from build123d import *

# Parameters (mm, degrees)
SKETCH2_W           = 25
SKETCH2_H           = 25
SKETCH2_R           = 9.247
BOSS_EXTRUDE1_DEPTH = 100
BOSS_EXTRUDE1_DRAFT = -0.05
FILLET4_R           = 2


with BuildPart() as part:
    # Sketch2 → Boss-Extrude1 (with draft: the straight prism first)
    with BuildSketch(Plane(origin=(0, 0, 0), x_dir=(1, 0, 0), z_dir=(0, 1, 0))):
        Rectangle(SKETCH2_W, SKETCH2_H)
        Circle(SKETCH2_R, mode=Mode.SUBTRACT)
    extrude(amount=BOSS_EXTRUDE1_DEPTH)
    # Boss-Extrude1: the draft: its side faces are tilted about the plane it starts from
    boss_extrude1_sides = [part.faces().sort_by_distance(p)[0] for p in [
        (-12.5, 50, 0),
        (0, 50, 12.5),
        (12.5, 50, 0),
        (0, 50, -12.5),
        (-9.247, 50, 0),
    ]]
    draft(boss_extrude1_sides, Plane(origin=(0, 0, 0), x_dir=(1, 0, 0), z_dir=(0, 1, 0)), BOSS_EXTRUDE1_DRAFT)

    # Fillet4
    fillet4_edges = [part.edges().sort_by_distance(p)[0] for p in [
        (0, 0, 12.5),
        (-12.5, 0, 0),
        (0, 0, -12.5),
        (12.5, 0, 0),
        (-12.543633242, 50, -12.543633242),
        (12.543633242, 50, -12.543633242),
    ]]
    fillet(fillet4_edges, radius=FILLET4_R)


solid = part.part
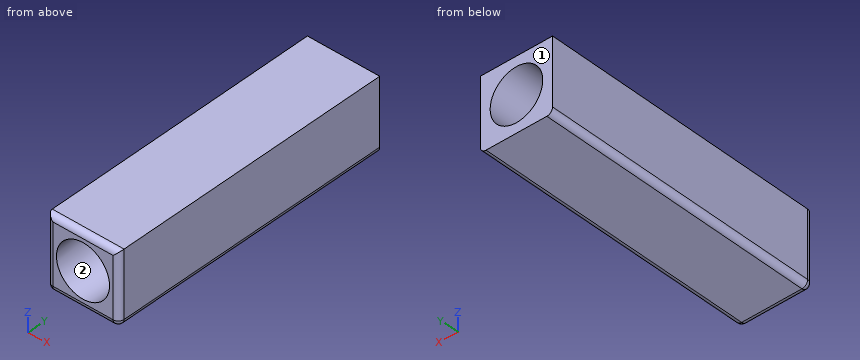
CAD build for the part. Positions are in the model's coordinates, mm. Face numbers are marked on the shaded views. Round coordinates to 2 decimals unless told otherwise and drop trailing zeros.
(1) Drop flat-ended pins along their axis: P1, Ø12, axis at x = -0.5, z = -2, coming from the +Y side; P2, Ø1.5, axis at y = 58.5, z = 2.5, coming from the +X side; P3, Ø1.5, axis at y = 49, z = -7, coming from the -X side; P4, Ø8, axis at x = -9, y = 25.5, coming from the -Z side. Give the stop position or say it passes through.
(2) Probe line 1 along X through (y, z) = (21, -10.5); line 2 along X through (y, z) = (16.5, -4.25); line 3 along X through (y, z) = (28, -0.5). List the from-to ranges inside material, lowest first.
(3) Mould opens along Z. For the marked faces 1 and 2 say: pulls with the +Z half, pulls with the -Z half, needs draft (parallel to the pull), parting line crosses it, or undercut.
From the geometry:
1. P1: passes through
1. P2: stops at x = 12.55
1. P3: stops at x = -12.54
1. P4: stops at z = -12.53
2. line 1: x = -12.52 to 12.52
2. line 2: x = -12.51 to -8.2, 8.2 to 12.51
2. line 3: x = -12.52 to -9.21, 9.21 to 12.52
3. face 1: needs draft
3. face 2: undercut
